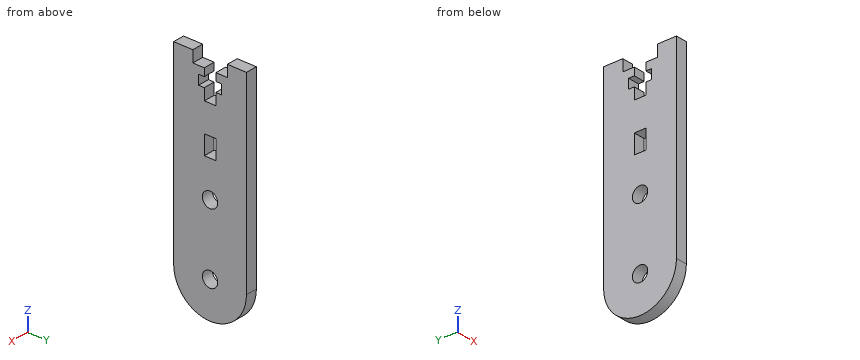
```python
from build123d import *

# Parameters (mm, degrees)
F0_R     = 2
F0_W     = 3
F0_H     = 5
F1_DEPTH = 3


with BuildPart() as f1:
    # F0 (on Right) → F1 (new body)
    with BuildSketch(Plane.YZ):
        with BuildLine():
            Line((-51.601472, 15.769853), (-56.601472, 15.769853))
            Line((-56.601472, 15.769853), (-56.601472, -34.680147))
            ThreePointArc((-56.601472, -34.680147), (-47.101472, -44.180147), (-37.601472, -34.680147))
            Line((-37.601472, -34.680147), (-37.601472, 15.769853))
            Line((-37.601472, 15.769853), (-42.601472, 15.769853))
            Line((-42.601472, 15.769853), (-42.601472, 12.769853))
            Line((-42.601472, 12.769853), (-45.601472, 12.769853))
            Line((-45.601472, 12.769853), (-45.601472, 10.769853))
            Line((-45.601472, 10.769853), (-44.101472, 10.769853))
            Line((-44.101472, 10.769853), (-44.101472, 8.269853))
            Line((-44.101472, 8.269853), (-45.601472, 8.269853))
            Line((-45.601472, 8.269853), (-45.601472, 5.269853))
            Line((-45.601472, 5.269853), (-48.601472, 5.269853))
            Line((-48.601472, 5.269853), (-48.601472, 8.269853))
            Line((-48.601472, 8.269853), (-50.101472, 8.269853))
            Line((-50.101472, 8.269853), (-50.101472, 10.769853))
            Line((-50.101472, 10.769853), (-48.601472, 10.769853))
            Line((-48.601472, 10.769853), (-48.601472, 12.769853))
            Line((-48.601472, 12.769853), (-51.601472, 12.769853))
            Line((-51.601472, 12.769853), (-51.601472, 15.769853))
        make_face()
        with Locations((-47.101472, -34.680147)):
            Circle(F0_R, mode=Mode.SUBTRACT)
        with Locations((-47.101472, -16.640147)):
            Circle(F0_R, mode=Mode.SUBTRACT)
        with Locations((-47.101472, -4.685147)):
            Rectangle(F0_W, F0_H, mode=Mode.SUBTRACT)
    extrude(amount=F1_DEPTH)


solid = f1.part
```
Model file for the job. Use its own axes, mm. Coordinates: 2 decimals unless noted, no trailing zeros. Order: outer loops, then holes, each group sorted by start corner. A loop starts at its lowest first (then second) coordinate and runs counter-clockwise, first axis right, second up. Notation, with made-up numbers: M 39,1.5 L 48,1.5 A14 ccw 48,12.5 Z; hole C 85.25,57 d7. An arc over 180 degrees is marked long. Answer as CSV lines item,"result".
(1) Flat gauge pins, fed straight in: pin 1 (3.5 mm diameter, centred on y = -47.1, z = -34.68, fed in from +X); pin 2 (4.5 mm diameter, centred on y = -47.1, z = -16.64, fed in from +X). Where does each tip first touch, or does it go through?
Geometry says:
pin 1,"passes through"
pin 2,"stops at x = 3"
(2) Band-saw the part on C-C, the plane x = 1.25. List the corners of the cut face in (y, z).
Geometry says:
outline,"M -56.6,-34.68 A9.5 ccw -37.6,-34.68 L -37.6,15.77 L -42.6,15.77 L -42.6,12.77 L -45.6,12.77 L -45.6,10.77 L -44.1,10.77 L -44.1,8.27 L -45.6,8.27 L -45.6,5.27 L -48.6,5.27 L -48.6,8.27 L -50.1,8.27 L -50.1,10.77 L -48.6,10.77 L -48.6,12.77 L -51.6,12.77 L -51.6,15.77 L -56.6,15.77 Z; hole C -47.1,-34.68 d4; hole C -47.1,-16.64 d4; hole M -48.6,-7.19 L -45.6,-7.19 L -45.6,-2.19 L -48.6,-2.19 Z"
(3) Band-saw the part on B-B, the plane y = -48. List the corners of the cut face in (x, z).
Geometry says:
outline,"M 0,-44.14 L 3,-44.14 L 3,-36.47 L 0,-36.47 Z; M 0,-32.89 L 3,-32.89 L 3,-18.43 L 0,-18.43 Z; M 0,-14.85 L 3,-14.85 L 3,-7.19 L 0,-7.19 Z; M 0,-2.19 L 3,-2.19 L 3,5.27 L 0,5.27 Z"
(4) Band-saw the part on A-A, the plane z = -3. List the corners of the cut face in (x, y), then the cut area to 3 significant figures.
Geometry says:
outline,"M 0,-56.6 L 3,-56.6 L 3,-48.6 L 0,-48.6 Z; M 0,-45.6 L 3,-45.6 L 3,-37.6 L 0,-37.6 Z"
area,"48.0 mm2"
(5) Band-saw the part on D-D, the plane y = -40.5. List the corners of the cut face in (x, z), then the cut area to 3 significant figures.
Geometry says:
outline,"M 0,-41.51 L 3,-41.51 L 3,15.77 L 0,15.77 Z"
area,"172 mm2"
(6) Wall check: line 1 along Y through (x, z) = (1.9, 6); line 2 along Z through (x, y) = (0.4, -46.25); line 3 along Y through (x, z) = (2.55, -34). Give the ranges that are in metal, low to high.
Geometry says:
line 1,"y = -56.6 to -48.6, -45.6 to -37.6"
line 2,"z = -44.14 to -36.49, -32.87 to -18.45, -14.83 to -7.19, -2.19 to 5.27"
line 3,"y = -56.6 to -48.98, -45.22 to -37.6"
